Part print with two shaded views. Sizes in mm from the minimum x, y, z corner. Round coordinates to 2 decimals unless told otherwise and drop trailing zeros. Loops run counter-clockwise (first coordinate to the right, second up) from the corner with the lowest first, then second, coordinate; pieces in that order, holes last.
(1) Cut at B-B on z = 31. List the corners of the cut face in (x, y), then the cut area to 3 significant figures.
(2) Probe probe 1 along Z at (x, y) = (5, 37.5) (1 decimal); probe 2 along Z at (x, y) = (0.75, 8); probe 3 along Y at (x, z) = (1.75, 37) (1 decimal). List the from-to ranges inside material, lowest first.
(3) Cut at A-A on y = 23.17. List the corners of the cut face in (x, z), then the cut area to 3 significant figures.
(4) Cut at D-D on x = 3.5. Count the separate pieces of the cut face and the enclosed holes in it, then the cut area to 4 significant figures.
(5) Mould opens along Z. For the marked faces 1, 2 and 3 say: +Z half, -Z half, draft (parallel to the pull), parting line (faces both ways), or undercut.
(6) Flat gauge pins, fed straight in: pin 1 (5 mm diameter, centred on y = 9.73, z = 30.31, fed in from +X); pin 2 (2 mm diameter, centred on x = 4.5, z = 71, fed in from +Y); pin 3 (2.5 mm diameter, centred on y = 36.61, z = 30.31, fed in from +X). Where does each tip first touch, or does it go through?
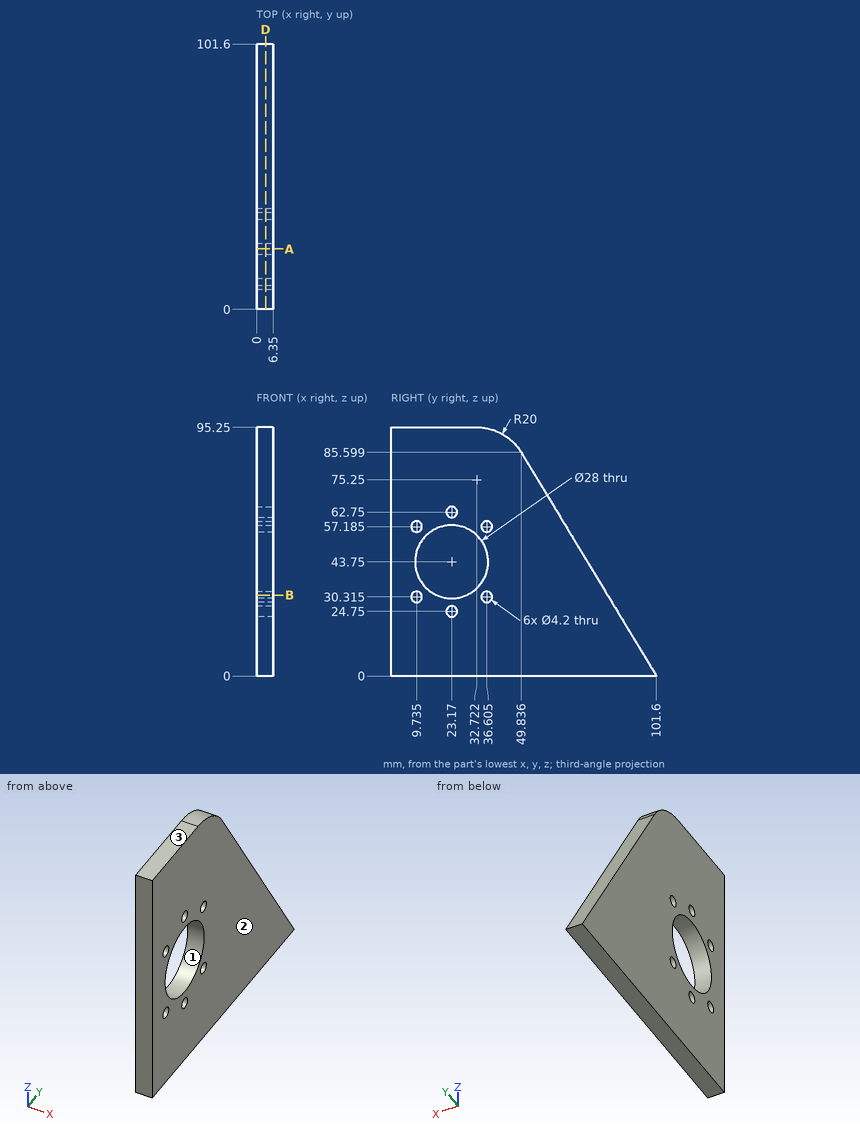
Final values:
1. outline: (0, 0) - (6.35, 0) - (6.35, 7.75) - (0, 7.75) - close; (0, 11.72) - (6.35, 11.72) - (6.35, 17.39) - (0, 17.39) - close; (0, 28.95) - (6.35, 28.95) - (6.35, 34.62) - (0, 34.62) - close; (0, 38.59) - (6.35, 38.59) - (6.35, 82.85) - (0, 82.85) - close
1. area: 402 mm2
2. probe 1: z = 0 to 28.4, 32.2 to 55.3, 59.1 to 94.7
2. probe 2: z = 0 to 29.13, 31.5 to 56, 58.37 to 95.25
2. probe 3: y = 0 to 10.9, 35.4 to 79.2
3. outline: (0, 0) - (6.35, 0) - (6.35, 22.65) - (0, 22.65) - close; (0, 26.85) - (6.35, 26.85) - (6.35, 29.75) - (0, 29.75) - close; (0, 57.75) - (6.35, 57.75) - (6.35, 60.65) - (0, 60.65) - close; (0, 64.85) - (6.35, 64.85) - (6.35, 95.25) - (0, 95.25) - close
3. area: 374 mm2
4. separate pieces: 1
4. enclosed holes: 7
4. area: 6,215 mm2
5. face 1: undercut
5. face 2: draft
5. face 3: +Z half
6. pin 1: stops at x = 6.35
6. pin 2: stops at y = 59.27
6. pin 3: passes through
